Model file for the job. Use its own axes, mm. A direction names the side the tool comes from. Coordinates: 2 decimals unless noted, no trailing zeros. Order: outer loops, then holes, each group sorted by start corner. A loop starts at its lowest first (then second) coordinate and runs counter-clockwise, first axis right, second up. Notation, with made-up numbers: (-24.5, 31.5) -> (6.5, 31.5) arc R7 ccw to (6.5, 36.5) -> close; hole circle Ø3 at (-3, 15.5). An arc over 180 degrees is marked (long way). Write item = value, one per line. Start each with the question number.
Q1. Cut at A-A, the plane z = 0. List the corners of the cut face in (x, y).
Q2. Flat gauge pins, fed straight in: pin 1 (6 mm diameter, centred on y = 5, z = -1, fed in from +X); pin 2 (3 mm diameter, centred on x = -50, y = 9, fed in from -Z); pin 3 (4 mm diameter, centred on x = -60, z = 0, fed in from +Y). Where does each tip first touch, or does it go through?
Q3. 3-axis set-ups, long thin cutter, end or side, ignore diameter. For faces 5 (the face through (4, 9, -3.2)), 6 (the face through (-8.44, 9.35, 6.06)): which of +Z, -Z, +X, -X, +Y, -Y reach the whole face in a straight line?
Q4. Cut at B-B, the plane x = -66.5. List the corners of the cut face in (y, z).
Q5. Mould opens along Y. For faces 1 (the face through (4, 5, 9)), 2 (the face through (68.414, 9.208, 6.059)), 3 (the face through (4, 4, 0)), 4 (the face through (-50.07, 10.6, 6.06)) say: +Y half, -Y half, draft (parallel to the pull), parting line (faces both ways), or undercut.
Q6. Wall check: line 1 (X direction, y = 9, z = -6.4); line 2 (X direction, y = 1.8, z = 0); line 3 (Y direction, x = 30, z = -6.5). Give the ranges that are in metal, low to high. Write a range as from..to.
Q7. Cut at C-C, the plane x = 60. List the corners of the cut face in (y, z).
Autodesk Inventor part; units mm, degrees
ref_plane "YZ Plane" through (0, 0, 0) normal (1, 0, 0) x (0, 1, 0)
ref_plane "XZ Plane" through (0, 0, 0) normal (0, 1, 0) x (-1, 0, 0)
ref_plane "XY Plane" through (0, 0, 0) normal (0, 0, 1) x (1, 0, 0)
sketch "スケッチ1" plane through (0, 0, 0) normal (0, 1, 0) x (-1, 0, 0)
  line L0 (-90, -3) -> (90, -3)
  line L1 (90, -3) -> (90, 3)
  line L2 (90, 3) -> (-90, 3)
  line L3 (-90, 3) -> (-90, -3)
  line L4 (-90, -3) -> (90, 3) construction
  line L5 (90, -3) -> (-90, 3) construction
  point P0 (0, 0)
  dimension "d0" = 180
  dimension "d1" = 6
extrude "押し出し1" add sketch "スケッチ1" along normal blind 17
sketch "スケッチ2" plane through (0, 0, 0) normal (0, -1, 0) x (1, 0, 0)
  line L0 (-90, 3) -> (90, 3)
  line L1 (90, 3) -> (-80, 3)
  line L2 (-80, 3) -> (-80, 9)
  line L3 (-80, 9) -> (90, 9)
  line L4 (90, 9) -> (90, 3)
  line L5 (90, 3) -> (90, -3)
  line L6 (90, -3) -> (-80, -3)
  line L7 (-80, -3) -> (-80, -6)
  line L8 (-80, -6) -> (90, -6)
  line L9 (90, -6) -> (90, -3)
  point P0 (0, 0)
  dimension "d4" = 170
  dimension "d5" = 6
  dimension "d6" = 170
  dimension "d7" = 3
extrude "押し出し2" add sketch "スケッチ2" against normal blind 14
sketch "スケッチ3" plane through (0, 17, 0) normal (0, 1, 0) x (1, 0, 0)
  line L0 (-90, 3) -> (-90, -3)
  line L1 (90, -3) -> (90, 3)
  line L2 (-90, 3) -> (90, 3)
  line L3 (90, 3) -> (90, -3)
  line L4 (90, -3) -> (-90, -3)
  line L5 (-90, -3) -> (-90, 3)
  point P0 (0, 0)
extrude "押し出し3" cut sketch "スケッチ3" against normal blind 13
sketch "スケッチ4" plane through (0, 4, 0) normal (0, 1, 0) x (1, 0, 0)
  line L0 (-90, -3) -> (-90, 3)
  line L1 (-80, 6) -> (-80, 3)
  line L2 (-90, -3) -> (-80, -3)
  line L3 (-80, -3) -> (-80, 3)
  line L4 (-80, 3) -> (-90, 3)
  line L5 (-90, 3) -> (-90, -3)
  point P0 (0, 0)
extrude "押し出し4" cut sketch "スケッチ4" against normal blind 13
sketch "スケッチ5" plane through (0, 14, 0) normal (0, 1, 0) x (1, 0, 0)
  line L0 (97.0492, -3.2) -> (-97.0492, -3.2)
  line L1 (-97.0492, -3.2) -> (-97.0492, 3.2)
  line L2 (-97.0492, 3.2) -> (97.0492, 3.2)
  line L3 (97.0492, 3.2) -> (97.0492, -3.2)
  line L4 (97.0492, -3.2) -> (-97.0492, 3.2) construction
  line L5 (-97.0492, -3.2) -> (97.0492, 3.2) construction
  point P0 (0, 0)
  dimension "d14" = 6.4
extrude "押し出し5" cut sketch "スケッチ5" against normal blind 10
sketch "スケッチ6" plane through (-80, 0, 9) normal (0, 0, 1) x (1, 0, 0)
  line L0 (0, 14) -> (170, 14)
  line L1 (170, 0) -> (170, 14)
  point P0 (80, 0)
  point P1 (150, 9)
  point P2 (110, 9)
  point P3 (70, 9)
  point P4 (30, 9)
  dimension "d17" = 5
  dimension "d18" = 20
  dimension "d19" = 40
  dimension "d20" = 5
  dimension "d21" = 40
  dimension "d22" = 40
hole "穴1" at (70, 9, 9) at (30, 9, 9) at (-10, 9, 9) at (-50, 9, 9) direction (0, 0, -1) diameter 3.2 end through all
sketch "スケッチ7" plane through (0, 0, 0) normal (0, -1, 0) x (1, 0, 0)
  line L0 (-80, -6) -> (90, -6)
  line L1 (90, -6) -> (90, 9)
  line L2 (-80, -3.2) -> (90, -3.2)
  point P0 (0, 0)
  point P1 (60, 0)
  point P2 (0, 0)
  point P3 (-60, 0)
  dimension "d30" = 6
  dimension "d31" = 30
  dimension "d32" = 60
hole "穴2" at (60, 0, 0) at (0, 0, 0) at (-60, 0, 0) direction (0, 1, 0) diameter 3.2 end through all
sketch "スケッチ8" plane through (90, 0, -6) normal (0, 0, -1) x (-1, 0, 0)
  line L0 (0, 0) -> (0, 14)
  line L1 (0, 0) -> (170, 0)
  line L2 (170, 0) -> (170, 14)
  line L3 (170, 14) -> (0, 14)
  line L4 (0, 14) -> (0, 0)
  point P0 (90, 0)
extrude "押し出し6" add sketch "スケッチ8" along normal blind 1
sketch "スケッチ9" plane through (90, 0, -7) normal (0, 0, -1) x (-1, 0, 0)
  circle A0 centre (20, 9) radius 1.6
  circle A1 centre (60, 9) radius 1.6
  circle A2 centre (100, 9) radius 1.6
  circle A3 centre (140, 9) radius 1.6
  point P0 (90, 0)
hole "穴3" at (70, 9, -7) at (30, 9, -7) at (-10, 9, -7) at (-50, 9, -7) direction (0, 0, 1) diameter 3.2 depth 10
sketch "スケッチ10" plane through (0, 0, 0) normal (0, -1, 0) x (1, 0, 0)
  line L0 (90, -7) -> (90, 9)
  line L1 (-80, 9) -> (90, 9)
  line L2 (90, -7) -> (-80, -7)
  line L3 (-80, -7) -> (-80, 9)
  line L4 (-80, 9) -> (90, 9)
  line L5 (90, 9) -> (90, -7)
  point P0 (0, 0)
extrude "押し出し7" add sketch "スケッチ10" along normal blind 5
sketch "スケッチ11" plane through (0, -5, 0) normal (0, -1, 0) x (1, 0, 0)
  circle A0 centre (0, 0) radius 1.6
  circle A1 centre (-60, 0) radius 1.6
  circle A2 centre (60, 0) radius 1.6
hole "穴4" at (0, -5, 0) at (-60, -5, 0) at (60, -5, 0) direction (0, 1, 0) diameter 3.2 depth 10
properties part number "lock1"
Here are the results:
q1.outline = (-80, -5) -> (-61.6, -5) -> (-61.6, 4) -> (-80, 4) -> close; (-58.4, -5) -> (-1.6, -5) -> (-1.6, 4) -> (-58.4, 4) -> close; (1.6, -5) -> (58.4, -5) -> (58.4, 4) -> (1.6, 4) -> close; (61.6, -5) -> (90, -5) -> (90, 4) -> (61.6, 4) -> close
q2.pin_1 = 90
q2.pin_2 = through
q2.pin_3 = 4
q3.face_5 = +X, -X, +Y
q3.face_6 = +Z, -Z
q4.outline = (-5, -7) -> (14, -7) -> (14, -3.2) -> (4, -3.2) -> (4, 3.2) -> (14, 3.2) -> (14, 9) -> (-5, 9) -> close
q5.face_1 = draft
q5.face_2 = undercut
q5.face_3 = +Y half
q5.face_4 = undercut
q6.line_1 = -80..-51.6, -48.4..-11.6, -8.4..28.4, 31.6..68.4, 71.6..90
q6.line_2 = -80..-61.6, -58.4..-1.6, 1.6..58.4, 61.6..90
q6.line_3 = -5..7.4, 10.6..14
q7.outline = (-5, -7) -> (14, -7) -> (14, -3.2) -> (4, -3.2) -> (4, -1.6) -> (-5, -1.6) -> close; (-5, 1.6) -> (4, 1.6) -> (4, 3.2) -> (14, 3.2) -> (14, 9) -> (-5, 9) -> close
